```python
from build123d import *

# Parameters (mm, degrees)
F0_R     = 9.525
F0_R_2   = 6.35
F1_DEPTH = 3.175
F2_DEPTH = 12.7
F3_DEPTH = 3.175


# Not quite as in the source:
# - a feature names something its author has since deleted; it is built from what else it names


with BuildPart() as f1:
    # F0 (on Top) → F1 (new body)
    with BuildSketch(Plane.XY):
        Polygon((0, 127), (0, 0), (127, 0), align=None)
        with Locations((33.6748659611, 33.6748659611)):
            Circle(F0_R, mode=Mode.SUBTRACT)
        Polygon((127, 0), (0, 0), (0, 127), (-3.175, 127), (-3.175, -3.175), (127, -3.175), align=None)
        with Locations((33.6748659611, 33.6748659611)):
            Circle(F0_R)
        with Locations((33.6748659611, 33.6748659611)):
            Circle(F0_R_2, mode=Mode.SUBTRACT)
    extrude(amount=F1_DEPTH)

    # F0 (on Top) → F2 (join)
    with BuildSketch(Plane.XY):
        Polygon((127, 0), (0, 0), (0, 127), (-3.175, 127), (-3.175, -3.175), (127, -3.175), align=None)
    extrude(amount=F2_DEPTH)

    # F0 (on Top) → F3 (join)
    with BuildSketch(Plane.XY):
        with Locations((33.6748659611, 33.6748659611)):
            Circle(F0_R)
        with Locations((33.6748659611, 33.6748659611)):
            Circle(F0_R_2, mode=Mode.SUBTRACT)
    extrude(amount=-F3_DEPTH)


solid = f1.part
```
Here's how the part is built. I have some questions about the finished solid (model axes, mm). A direction names the side the tool comes from. Give positions to 0.01 mm unless a question says otherwise; leave off trailing zeros. Loops run counter-clockwise (first coordinate to the right, second up) from the corner with the lowest first, then second, coordinate; pieces in that order, holes last. Notation, with made-up numbers: M 20.25,37 L 64.25,37 A15 ccw 64.25,46 Z; hole C 46,-28 d7. An arc over 180 degrees is marked long. Put each result on its own line as item: value. Start each with the question number.
(1) Will these pins go through, and if not, where does the flat tip stop? pin 1 Ø3 at (y, z) = (27.5, 11) entering from +X; pin 2 Ø1 at (x, y) = (48.5, 11.5) entering from +Z (3 decimals); pin 3 Ø5 at (x, z) = (34, 7.5) entering from +Y.
(2) I want a section at C-C on z = 4.75. Please give me the cut outline in (x, y) (3 decimals).
(3) I want a section at A-A on x = 30. Please give me the cut outline in (y, z) (3 decimals).
(4) I need wall thicknesses on line 1 along Y through (x, z) = (65.5, 11) (3 decimals); line 2 along Z through (x, y) = (55.5, 13.5) (3 decimals). Which ranges of each line are inside material? Lowest first, please. Write a range as [from, to].
(5) I want a section at B-B on y = 99. Please give me the cut outline in (x, z) (3 decimals), then the cut area to 3 significant figures.
(6) For faces 1 (the cylindrical face through (38.07, 25.225, -1.565)), 2 (the flat face through (0, 63, 8)), 3 (the flat face through (127, -2, 6)), which set-ups out of +Z, -Z, +X, -X, +Y, -Y let a thin tool reach every point of the face, with its end or its side?
Answer block:
1. pin 1: x = 0
1. pin 2: z = 3.175
1. pin 3: y = 0
2. outline: M -3.175,-3.175 L 127,-3.175 L 127,0 L 0,0 L 0,127 L -3.175,127 Z
3. outline: M -3.175,0 L 24.887,0 L 24.887,-3.175 L 28.496,-3.175 L 28.496,3.175 L 0,3.175 L 0,12.7 L -3.175,12.7 Z; M 38.853,-3.175 L 42.462,-3.175 L 42.462,0 L 97,0 L 97,3.175 L 38.853,3.175 Z
4. line 1: [-3.175, 0]
4. line 2: [0, 3.175]
5. outline: M -3.175,0 L 28,0 L 28,3.175 L 0,3.175 L 0,12.7 L -3.175,12.7 Z
5. area: 129 mm^2
6. face 1: -Z
6. face 2: +Z, +X, +Y
6. face 3: +Z, -Z, +X, +Y, -Y
